Model file for the job. Use its own axes, mm. Round coordinates to 2 decimals unless told otherwise and drop trailing zeros. Order: outer loops, then holes, each group sorted by start corner. A loop starts at its lowest first (then second) coordinate and runs counter-clockwise, first axis right, second up. Notation, with made-up numbers: (21.25, -22) - (68.25, -22) arc R8 ccw to (68.25, -17) - close; hole circle Ø4 at (14.5, -24.75). An arc over 180 degrees is marked (long way). Write item = value, one per line. Start each with the question number.
from build123d import *

# Parameters (mm, degrees)
SKETCH1_R           = 6.439788541
BOSS_EXTRUDE3_DEPTH = 93.98


with BuildPart() as part:
    # Sketch1 → Boss-Extrude3 (new body)
    with BuildSketch(Plane.XY):
        with BuildLine():
            Line((-88.871195362, 30.911720126), (57.437556069, 30.911720126))
            ThreePointArc((57.437556069, 30.911720126), (64.778520858, 27.870992949), (67.819248035, 20.53002816))
            Line((67.819248035, 20.53002816), (67.819248035, 0.255438821))
            ThreePointArc((67.819248035, 0.255438821), (64.778520858, -7.085525968), (57.437556069, -10.126253145))
            Line((57.437556069, -10.126253145), (-88.327193145, -10.126253145))
            ThreePointArc((-88.327193145, -10.126253145), (-94.733815173, -7.472543412), (-97.387524906, -1.065921384))
            Line((-97.387524906, -1.065921384), (-97.387524906, 22.395390582))
            Line((-97.387524906, 22.395390582), (-88.871195362, 30.911720126))
        make_face()
        with Locations((-86.472872248, 0)):
            Circle(SKETCH1_R, mode=Mode.SUBTRACT)
        with Locations((46.939064733, 0)):
            Circle(SKETCH1_R, mode=Mode.SUBTRACT)
    extrude(amount=-BOSS_EXTRUDE3_DEPTH)


solid = part.part
Item 1: Saw through at B-B, the plane y = -3. Give the cut face in (x, z).
Item 2: Mould opens along Y. For faces 1 (the face through (-94.663, -7.543, -46.332)), 2 (the face through (-17, 30.912, -46)), 3 (the face through (-80.524, -2.466, -46.332)) say: +Y half, -Y half, draft (parallel to the pull), parting line (faces both ways), or undercut.
Item 3: Probe L1, parallel to X at y = -2.5, z = -84.5; L2, parallel to Y at x = -88, z = -72; L3, parallel to X at y = 5, z = -47.5. List the from-to ranges inside material, lowest first.
Item 4: Saw through at A-A, the plane z = -51. Give the cut face in (x, y), then the cut area to 3 significant figures.
Item 5: Drop flat-ended pins along their axis: pin 1 (1.5 mm diameter, centred on y = -1, z = -26, fed in from +X); pin 2 (11.5 mm diameter, centred on x = 46.94, y = 0, fed in from -Z). Give the stop position or say it passes through.
Check sheet entries:
q1.outline = (-97.18, -93.98) - (-92.17, -93.98) - (-92.17, 0) - (-97.18, 0) - close; (-80.77, -93.98) - (41.24, -93.98) - (41.24, 0) - (-80.77, 0) - close; (52.64, -93.98) - (67.3, -93.98) - (67.3, 0) - (52.64, 0) - close
q2.face_1 = -Y half
q2.face_2 = +Y half
q2.face_3 = undercut
q3.L1 = -97.27 to -92.41, -80.54 to 41, 52.87 to 67.45
q3.L2 = -10.13 to -6.26, 6.26 to 30.91
q3.L3 = -97.39 to -90.53, -82.41 to 42.88, 51 to 67.82
q4.outline = (-97.39, -1.07) arc R9.06 ccw to (-88.33, -10.13) - (57.44, -10.13) arc R10.38 ccw to (67.82, 0.26) - (67.82, 20.53) arc R10.38 ccw to (57.44, 30.91) - (-88.87, 30.91) - (-97.39, 22.4) - close; hole circle Ø12.88 at (-86.47, 0); hole circle Ø12.88 at (46.94, 0)
q4.area = 6,420 mm2
q5.pin_1 = 67.81
q5.pin_2 = through
